The listing builds one solid part. Answer for the finished solid, in the listing's coordinates (mm). Face numbers are marked on the shaded views. Give positions to 0.01 mm unless a question says otherwise; leave off trailing zeros. Write each loop counter-clockwise with the first axis right and the second up, starting at its lowest first coordinate (ties: lowest second). Pieces come first, ordered by that corner, then holes. Notation, with made-up numbers: (55, 42) - (82, 42) arc R7 ccw to (82, 53) - close; hole circle Ø10 at (45.5, 16). An arc over 180 degrees is marked (long way). Answer in a Markdown table with one row per item. Add a question column.
from build123d import *

# Parameters (mm, degrees)
F0_R     = 7.9375
F0_R_2   = 4.7625
F1_DEPTH = 6.35
F3_R     = 1.7526
F4_DEPTH = 5.08
F5_SIZE  = 0.635


with BuildPart() as f1:
    # F0 (on Top) → F1 (new body)
    with BuildSketch(Plane.XY):
        Circle(F0_R)
        Circle(F0_R_2, mode=Mode.SUBTRACT)
    extrude(amount=F1_DEPTH)

    # F3 (on offset) → F4 (cut)
    with BuildSketch(Plane.YZ.offset(7.9375)):
        with Locations((0, 3.175)):
            Circle(F3_R)
    extrude(amount=-F4_DEPTH, mode=Mode.SUBTRACT)

    # F5
    f5_edges = [f1.edges().sort_by_distance(p)[0] for p in [
        (-7.9375, 0, 6.35),
        (-7.9375, 0, 0),
    ]]
    chamfer(f5_edges, length=F5_SIZE)


solid = f1.part
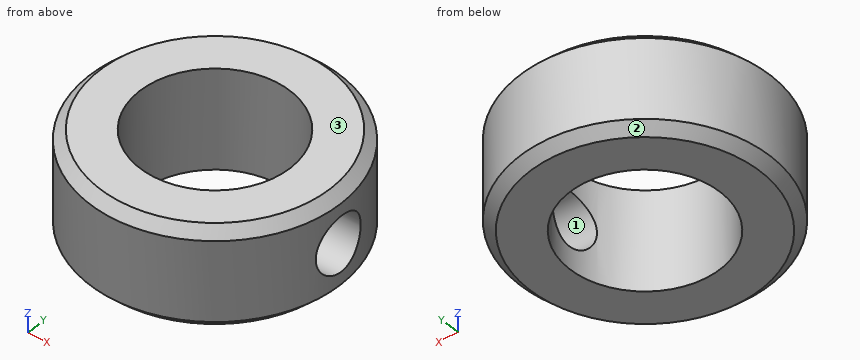
1. Straight lines are drawn through the part: L1, parallel to Y at x = 0, z = 2.25; L2, parallel to X at y = 2.75, z = 2.75; L3, parallel to Z at x = 6.25, y = 0. For each, find the intervals that lie inside material, in ascending order. Write a range as [from, to].
2. The mould has two halves that part along Y. Classify the marked faces 1, 2 and 3: +Y half, -Y half, draft (parallel to the pull), parting line (faces both ways), or undercut.
3. Section C-C (z = 4.5) is taken. Give the vertices of the cut face in (x, y) (1 decimal), and give its area (3 significant figures).
4. Given pin 1 Ø2 at (x, z) = (-4, 3) entering from +Y, flat-ended and moving along its own axis, determine where the tip first touches the part or whether it passes through.
5. Section A-A (y = 0) is taken. State how many separate pieces and enclosed holes the cut face has, and give its area (3 significant figures).
Geometry check:
| question | item | result |
|---|---|---|
| 1 | L1 | [-7.94, -4.76], [4.76, 7.94] |
| 1 | L2 | [-7.45, -3.89], [3.89, 7.45] |
| 1 | L3 | [0, 1.42], [4.93, 6.35] |
| 2 | face 1 | undercut |
| 2 | face 2 | parting line |
| 2 | face 3 | draft |
| 3 | outline | (4.6, -1.1) arc R4.8 cw (long way) to (4.6, 1.1) - (7.9, 1.1) arc R7.9 ccw (long way) to (7.9, -1.1) - close |
| 3 | area | 119 mm² |
| 4 | pin 1 | y = 7.35 |
| 5 | separate pieces | 3 |
| 5 | enclosed holes | 0 |
| 5 | area | 28.4 mm² |
